```python
from build123d import *

# Parameters (mm, degrees)
BOSS_EXTRUDE1_DEPTH = 3.175
SKETCH2_R           = 2.5796875
CUT_EXTRUDE1_DEPTH  = 3.175
FILLET1_R           = 2.54


with BuildPart() as part:
    # Sketch1 → Boss-Extrude1 (new body)
    with BuildSketch(Plane.XY):
        Polygon((-12.7, -63.5), (12.7, -63.5), (12.7, 12.7), (63.5, 12.7), (63.5, 63.5), (12.7, 63.5), (-12.7, 63.5), align=None)
    extrude(amount=BOSS_EXTRUDE1_DEPTH)

    # Sketch2 → Cut-Extrude1 (cut)
    with BuildSketch(Plane.XY.offset(3.175)):
        with Locations((0, 38.1)):
            Circle(SKETCH2_R)
        with Locations((38.1, 38.1)):
            Circle(SKETCH2_R)
        with Locations((0, -38.1)):
            Circle(SKETCH2_R)
        with Locations((0, -12.7)):
            Circle(SKETCH2_R)
    extrude(amount=-CUT_EXTRUDE1_DEPTH, mode=Mode.SUBTRACT)

    # Fillet1
    fillet1_edges = [part.edges().sort_by_distance(p)[0] for p in [
        (63.5, 63.5, 1.5875),
        (63.5, 12.7, 1.5875),
        (12.7, 12.7, 1.5875),
        (12.7, -63.5, 1.5875),
        (-12.7, -63.5, 1.5875),
        (-12.7, 63.5, 1.5875),
    ]]
    fillet(fillet1_edges, radius=FILLET1_R)


solid = part.part
```
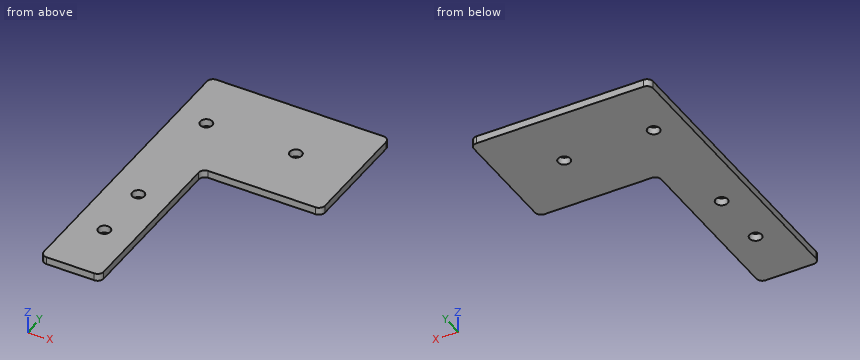
Design review of the part built by this model. Coordinates are the model's own, in mm. Give positions to 0.01 mm unless a question says otherwise; leave off trailing zeros. Write each loop counter-clockwise with the first axis right and the second up, starting at its lowest first coordinate (ties: lowest second). Pieces come first, ordered by that corner, then holes.
(1) Add section A-A (x = 0). Give the boundary of the cut face in (y, z) (3 decimals).
Checked values:
outline: (-63.5, 0) - (-40.68, 0) - (-40.68, 3.175) - (-63.5, 3.175) - close; (-35.52, 0) - (-15.28, 0) - (-15.28, 3.175) - (-35.52, 3.175) - close; (-10.12, 0) - (35.52, 0) - (35.52, 3.175) - (-10.12, 3.175) - close; (40.68, 0) - (63.5, 0) - (63.5, 3.175) - (40.68, 3.175) - close
(2) Add section D-D (z = 2.45). Give the boundary of the cut face in (x, y), and give its area (3 significant figures).
Checked values:
outline: (-12.7, -60.96) arc R2.54 ccw to (-10.16, -63.5) - (10.16, -63.5) arc R2.54 ccw to (12.7, -60.96) - (12.7, 10.16) arc R2.54 cw to (15.24, 12.7) - (60.96, 12.7) arc R2.54 ccw to (63.5, 15.24) - (63.5, 60.96) arc R2.54 ccw to (60.96, 63.5) - (-10.16, 63.5) arc R2.54 ccw to (-12.7, 60.96) - close; hole circle Ø5.16 at (0, -38.1); hole circle Ø5.16 at (0, -12.7); hole circle Ø5.16 at (0, 38.1); hole circle Ø5.16 at (38.1, 38.1)
area: 5,720 mm2
(3) Add section B-B (y = 38.1). Give the boundary of the cut face in (x, z) (3 decimals).
Checked values:
outline: (-12.7, 0) - (-2.58, 0) - (-2.58, 3.175) - (-12.7, 3.175) - close; (2.58, 0) - (35.52, 0) - (35.52, 3.175) - (2.58, 3.175) - close; (40.68, 0) - (63.5, 0) - (63.5, 3.175) - (40.68, 3.175) - close
(4) Add section C-C (y = -38.1). Give the boundary of the cut face in (x, z) (3 decimals), and give its area (3 significant figures).
Checked values:
outline: (-12.7, 0) - (-2.58, 0) - (-2.58, 3.175) - (-12.7, 3.175) - close; (2.58, 0) - (12.7, 0) - (12.7, 3.175) - (2.58, 3.175) - close
area: 64.3 mm2
(5) Wall thickness on line 1 along Y through (x, z) = (0, 2.45); line 2 along Y through (x, z) = (38.1, 1.2); line 3 along X through (y, z) = (-43.5, 0.9): over which ranges is each line inside the solid? List them lowest first.
Checked values:
line 1: y = -63.5 to -40.68, -35.52 to -15.28, -10.12 to 35.52, 40.68 to 63.5
line 2: y = 12.7 to 35.52, 40.68 to 63.5
line 3: x = -12.7 to 12.7
(6) Clearance check with flat-ended pins moving along their axes: pin 1 Ø4 at (x, y) = (0, 38.1) entering from +Z; pin 2 Ø1 at (x, z) = (42.5, 1) entering from -Y; pin 3 Ø1.6 at (y, z) = (-29, 2.5) entering from +X. State where each tip first meets the part, or that it passes through.
Checked values:
pin 1: passes through
pin 2: stops at y = 12.7
pin 3: stops at x = 12.7
